```python
from build123d import *

# Parameters (mm, degrees)
BOSS_EXTRUDE3_DEPTH = 71.12
FILLET3_R           = 35.56
SKETCH6_R           = 6.35
CUT_EXTRUDE1_DEPTH  = 154.603584906


with BuildPart() as part:
    # Sketch1 → Boss-Extrude3 (new body)
    with BuildSketch(Plane.XY):
        with BuildLine():
            Line((-144.822728972, 103.115454206), (-144.822728972, -16.264545794))
            ThreePointArc((-144.822728972, -16.264545794), (-141.102985093, -25.244801915), (-132.122728972, -28.964545794))
            Line((-132.122728972, -28.964545794), (-68.622728972, -28.964545794))
            ThreePointArc((-68.622728972, -28.964545794), (-59.642472851, -25.244801915), (-55.922728972, -16.264545794))
            Line((-55.922728972, -16.264545794), (-55.922728972, 103.115454206))
            Line((-55.922728972, 103.115454206), (-63.872928972, 103.115454206))
            Line((-63.872928972, 103.115454206), (-63.872928972, -16.264545794))
            ThreePointArc((-63.872928972, -16.264545794), (-65.264113183, -19.623161584), (-68.622728972, -21.014345794))
            Line((-68.622728972, -21.014345794), (-132.122728972, -21.014345794))
            ThreePointArc((-132.122728972, -21.014345794), (-135.481344761, -19.623161584), (-136.872528972, -16.264545794))
            Line((-136.872528972, -16.264545794), (-136.872528972, 103.115454206))
            Line((-136.872528972, 103.115454206), (-144.822728972, 103.115454206))
        make_face()
    extrude(amount=BOSS_EXTRUDE3_DEPTH)

    # Fillet3
    fillet3_edges = [part.edges().sort_by_distance(p)[0] for p in [
        (-59.897828972, 103.115454206, 71.12),
        (-59.897828972, 103.115454206, 0),
        (-140.847628972, 103.115454206, 0),
        (-140.847628972, 103.115454206, 71.12),
    ]]
    fillet(fillet3_edges, radius=FILLET3_R - 0.0001)  # a hair under: the kernel refuses the full size

    # Sketch6 → Cut-Extrude1 (cut, through all)
    with BuildSketch(Plane(origin=(-55.922728972, 0, 0), x_dir=(0, 0, -1), z_dir=(1, 0, 0))):
        with Locations((-35.56, 67.555454206)):
            Circle(SKETCH6_R)
    extrude(amount=-CUT_EXTRUDE1_DEPTH, mode=Mode.SUBTRACT)


solid = part.part
```
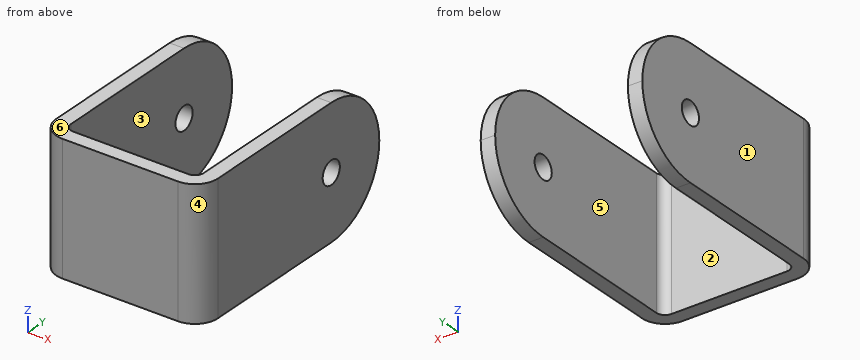
Build history of the part. All positions in model axes, mm. Face numbers are marked on the shaded views. A direction names the side the tool comes from. Round coordinates to 2 decimals unless told otherwise and drop trailing zeros. Write each loop counter-clockwise with the first axis right and the second up, starting at its lowest first coordinate (ties: lowest second). Pieces come first, ordered by that corner, then holes.
1) Band-saw the part on D-D, the plane x = -89. List the corners of the cut face in (y, z).
2) Band-saw the part on C-C, the plane z = 59. List the corners of the cut face in (x, y), and give its area (3 significant figures).
3) Mould opens along X. For the marked faces 3, 4, 5 and 6 say: +X half, -X half, draft (parallel to the pull), parting line (faces both ways), or undercut.
4) 3-axis set-ups, long thin cutter, end or side, ignore diameter. For the marked faces 1 and 2: which of +Z, -Z, +X, -X, +Y, -Y reach the whole face in a straight line?
5) Pin check, flat tip, straight feed: pin 1 (10 mm diameter, centred on x = -68.5, z = 26.5, fed in from +Y). Stop position of the tip, or through.
6) Band-saw the part on A-A, the plane y = -9. List the corners of the cut face in (x, z), and give its area (3 significant figures).
7) Drill centre lines: probe 1 along X at (y, z) = (71, 10.5); probe 2 along Y at (x, z) = (-139, 35.56); probe 3 along Y at (x, z) = (-142, 35). Where is each one in solid material? Low to high.
8) Band-saw the part on B-B, the plane y = 71.5. List the corners of the cut face in (x, z).
Ans:
1. outline: (-28.96, 0) - (-21.01, 0) - (-21.01, 71.12) - (-28.96, 71.12) - close
2. outline: (-144.82, -16.26) arc R12.7 ccw to (-132.12, -28.96) - (-68.62, -28.96) arc R12.7 ccw to (-55.92, -16.26) - (-55.92, 94.3) - (-63.87, 94.3) - (-63.87, -16.26) arc R4.75 cw to (-68.62, -21.01) - (-132.12, -21.01) arc R4.75 cw to (-136.87, -16.26) - (-136.87, 94.3) - (-144.82, 94.3) - close
2. area: 2,480 mm2
3. face 3: undercut
3. face 4: +X half
3. face 5: undercut
3. face 6: draft
4. face 1: +Z, -Z, -X, +Y, -Y
4. face 2: +Z, -Z, +Y
5. pin 1: stops at y = 102.39
6. outline: (-144.82, 0) - (-136.87, 0) - (-136.87, 71.12) - (-144.82, 71.12) - close; (-63.87, 0) - (-55.92, 0) - (-55.92, 71.12) - (-63.87, 71.12) - close
6. area: 1,130 mm2
7. probe 1: x = -144.82 to -136.87, -63.87 to -55.92
7. probe 2: y = -26.94 to 61.21, 73.91 to 103.12
7. probe 3: y = -24.25 to 61.23, 73.88 to 103.11
8. outline: (-144.82, 0.22) - (-136.87, 0.22) - (-136.87, 30.58) - (-144.82, 30.58) - close; (-144.82, 40.54) - (-136.87, 40.54) - (-136.87, 70.9) - (-144.82, 70.9) - close; (-63.87, 0.22) - (-55.92, 0.22) - (-55.92, 30.58) - (-63.87, 30.58) - close; (-63.87, 40.54) - (-55.92, 40.54) - (-55.92, 70.9) - (-63.87, 70.9) - close
